Work out the finished part from the listing and answer in its coordinate system (mm). A direction names the side the tool comes from. Give positions to 0.01 mm unless a question says otherwise; leave off trailing zeros. Write each loop counter-clockwise with the first axis right and the second up, starting at its lowest first coordinate (ties: lowest second). Pieces come first, ordered by that corner, then holes.
1) Find section C-C (x = 9.5). Determine the outline of the cut face in (y, z), plus the area to 3 significant figures.
2) Find section D-D (y = 7). Determine the outline of the cut face in (x, z).
3) Determine the mould class of faces 3 (the face through (7.794, -1.308, 3.269)), 4 (the face through (22.4, 7.1, 3.9)), 5 (the face through (0, 0, 7.9)) for opening direction X: pulls with the +X half, pulls with the -X half, needs draft (parallel to the pull), parting line crosses it, or undercut.
4) Straight lines are drawn through the part: probe 1 along X at (y, z) = (-2, 7.25); probe 2 along X at (y, z) = (-1, 6.5); probe 3 along Y at (x, z) = (0, 1.75). For each, find the intervals that lie inside material, in ascending order.
5) Given pin 1 Ø1.5 at (y, z) = (-13, 3) entering from +X; pin 2 Ø5.5 at (x, y) = (-9.5, 0) entering from +Z, each flat-ended and moving along its own axis, determine where each tip first touches the part or whether it passes through.
6) Find section B-B (z = 1.25). Determine the outline of the cut face in (x, y).
7) A tool of negligible diameter and unlimited length cuts with its end or side. For faces 1 (the face through (-13.296, 0.167, 7.654)), 2 (the face through (0, 0, 0)), from which of +Z, -Z, +X, -X, +Y, -Y can it reach the whole face along a straight path? Write none if from no direction.
8) Find section A-A (y = 0). Determine the outline of the cut face in (x, z), plus the area to 3 significant figures.
```python
from build123d import *

# Parameters (mm, degrees)
SKETCH1_R           = 23.5
BOSS_EXTRUDE1_DEPTH = 7.9
CUT_EXTRUDE1_REACH  = 36.16
SKETCH2_R           = 2.15
SKETCH3_R           = 3.8
CUT_EXTRUDE2_DEPTH  = 0.5


with BuildPart() as part:
    # Sketch1 → Boss-Extrude1 (new body)
    with BuildSketch(Plane.XY):
        Circle(SKETCH1_R)
    extrude(amount=BOSS_EXTRUDE1_DEPTH)

    # Sketch2 → Cut-Extrude1 (cut, up to next)
    with BuildSketch(Plane.XY.offset(7.9), mode=Mode.PRIVATE) as cut_extrude1_sk1:
        with Locations((-9.5, 0)):
            Circle(SKETCH2_R)
    cut_extrude1_tool1 = extrude(cut_extrude1_sk1.sketch, amount=-CUT_EXTRUDE1_REACH, mode=Mode.PRIVATE) & part.part
    # Sketch2 → Cut-Extrude1 (cut, up to next)
    with BuildSketch(Plane.XY.offset(7.9), mode=Mode.PRIVATE) as cut_extrude1_sk2:
        with Locations((9.5, 0)):
            Circle(SKETCH2_R)
    cut_extrude1_tool2 = extrude(cut_extrude1_sk2.sketch, amount=-CUT_EXTRUDE1_REACH, mode=Mode.PRIVATE) & part.part
    add(cut_extrude1_tool1.solids().sort_by_distance((-9.5, 0, 7.9))[0], mode=Mode.SUBTRACT)
    add(cut_extrude1_tool2.solids().sort_by_distance((9.5, 0, 7.9))[0], mode=Mode.SUBTRACT)

    # Sketch3 → Cut-Extrude2 (cut)
    with BuildSketch(Plane.XY.offset(7.9)):
        with Locations((-9.5, 0)):
            Circle(SKETCH3_R)
        with Locations((9.5, 0)):
            Circle(SKETCH3_R)
    extrude(amount=-CUT_EXTRUDE2_DEPTH, mode=Mode.SUBTRACT)

    # Sketch7 → Cut-Revolve5 (revolve, cut)
    with BuildSketch(Plane(origin=(0, 0, 0), x_dir=(1, 0, 0), z_dir=(0, 1, 0)), mode=Mode.PRIVATE) as cut_revolve5_sk:
        Polygon((9.5, -7.4), (9.5, -5.206068977), (5.7, -7.4), align=None)
    revolve(cut_revolve5_sk.sketch.rotate(Axis((9.5, 0, 7.4), (0, 0, -1)), 180), axis=Axis((9.5, 0, 7.4), (0, 0, -1)), mode=Mode.SUBTRACT)

    # Sketch6 → Cut-Revolve6 (revolve, cut)
    with BuildSketch(Plane(origin=(0, 0, 0), x_dir=(1, 0, 0), z_dir=(0, 1, 0)), mode=Mode.PRIVATE) as cut_revolve6_sk:
        Polygon((-9.5, -7.4), (-9.5, -5.206068977), (-13.3, -7.4), align=None)
    revolve(cut_revolve6_sk.sketch.rotate(Axis((-9.5, 0, 7.4), (0, 0, -1)), 180), axis=Axis((-9.5, 0, 7.4), (0, 0, -1)), mode=Mode.SUBTRACT)


solid = part.part
```
Results:
1. outline: (-21.49, 0) - (-2.15, 0) - (-2.15, 6.45) - (-3.8, 7.4) - (-3.8, 7.9) - (-21.49, 7.9) - close; (2.15, 0) - (21.49, 0) - (21.49, 7.9) - (3.8, 7.9) - (3.8, 7.4) - (2.15, 6.45) - close
1. area: 302 mm2
2. outline: (-22.43, 0) - (22.43, 0) - (22.43, 7.9) - (-22.43, 7.9) - close
3. face 3: undercut
3. face 4: parting line crosses it
3. face 5: needs draft
4. probe 1: x = -23.41 to -12.42, -6.58 to 6.58, 12.42 to 23.41
4. probe 2: x = -23.48 to -11.51, -7.49 to 7.49, 11.51 to 23.48
4. probe 3: y = -23.5 to 23.5
5. pin 1: stops at x = 20.05
5. pin 2: stops at z = 6.79
6. outline: circle Ø47 at (0, 0); hole circle Ø4.3 at (-9.5, 0); hole circle Ø4.3 at (9.5, 0)
7. face 1: +Z
7. face 2: -Z, +X, -X, +Y, -Y
8. outline: (-23.5, 0) - (-11.65, 0) - (-11.65, 6.45) - (-13.3, 7.4) - (-13.3, 7.9) - (-23.5, 7.9) - close; (-7.35, 0) - (7.35, 0) - (7.35, 6.45) - (5.7, 7.4) - (5.7, 7.9) - (-5.7, 7.9) - (-5.7, 7.4) - (-7.35, 6.45) - close; (11.65, 0) - (23.5, 0) - (23.5, 7.9) - (13.3, 7.9) - (13.3, 7.4) - (11.65, 6.45) - close
8. area: 297 mm2
